Design review of the part built by this model. Coordinates are the model's own, in mm. Coordinates: 2 decimals unless noted, no trailing zeros. Write each loop counter-clockwise with the first axis right and the second up, starting at its lowest first coordinate (ties: lowest second). Pieces come first, ordered by that corner, then holes.
Q1. Add section A-A, the plane x = 0. Give the boundary of the cut face in (y, z), plus the area to 3 significant figures.
Q2. Add section C-C, the plane y = 3. Give the number of separate pieces and of enclosed holes in the cut face, plus the area to 3 significant figures.
Q3. Add section B-B, the plane z = 0. Give the boundary of the cut face in (x, y).
Q4. To check wall thickness, follow probe 1 along X at (y, z) = (4.25, 0); probe 2 along Z at (x, y) = (0, 5.75); probe 3 along Z at (x, y) = (42.5, 4.25). State the ranges of each line that lie inside material, in increasing order.
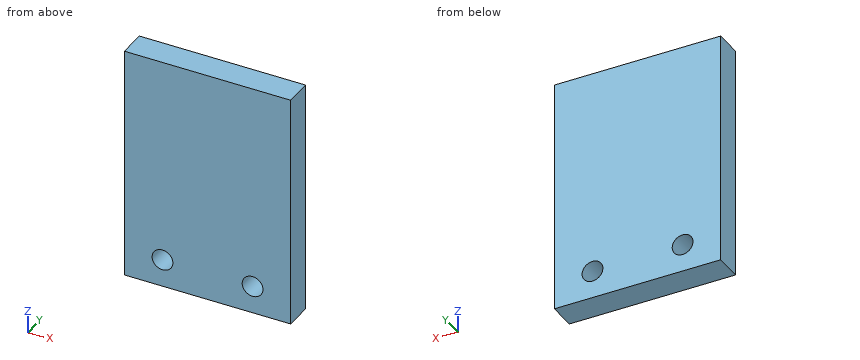
from build123d import *

# Parameters (mm, degrees)
SKETCH1_W           = 76.2
SKETCH1_H           = 107.95
SKETCH1_R           = 4.7625
BOSS_EXTRUDE1_DEPTH = 12.7


with BuildPart() as part:
    # Sketch1 → Boss-Extrude1 (new body)
    with BuildSketch(Plane(origin=(0, 0, 0), x_dir=(1, 0, 0), z_dir=(0, 1, 0))):
        with Locations((20.6375, -41.275)):
            Rectangle(SKETCH1_W, SKETCH1_H)
        Circle(SKETCH1_R, mode=Mode.SUBTRACT)
        with Locations((41.275, 0)):
            Circle(SKETCH1_R, mode=Mode.SUBTRACT)
    extrude(amount=BOSS_EXTRUDE1_DEPTH)


solid = part.part
Here are the results:
1. outline: (0, -12.7) - (12.7, -12.7) - (12.7, -4.76) - (0, -4.76) - close; (0, 4.76) - (12.7, 4.76) - (12.7, 95.25) - (0, 95.25) - close
1. area: 1,250 mm2
2. separate pieces: 1
2. enclosed holes: 2
2. area: 8,080 mm2
3. outline: (-17.46, 0) - (-4.76, 0) - (-4.76, 12.7) - (-17.46, 12.7) - close; (4.76, 0) - (36.51, 0) - (36.51, 12.7) - (4.76, 12.7) - close; (46.04, 0) - (58.74, 0) - (58.74, 12.7) - (46.04, 12.7) - close
4. probe 1: x = -17.46 to -4.76, 4.76 to 36.51, 46.04 to 58.74
4. probe 2: z = -12.7 to -4.76, 4.76 to 95.25
4. probe 3: z = -12.7 to -4.6, 4.6 to 95.25
